Job drawing, mm, ordinate dimensions from the low corner. One solid piece. A direction names the side the tool comes from. Coordinates: 2 decimals unless noted, no trailing zeros. Write each loop counter-clockwise with the first axis right and the second up, starting at its lowest first coordinate (ties: lowest second). Pieces come first, ordered by that corner, then holes.
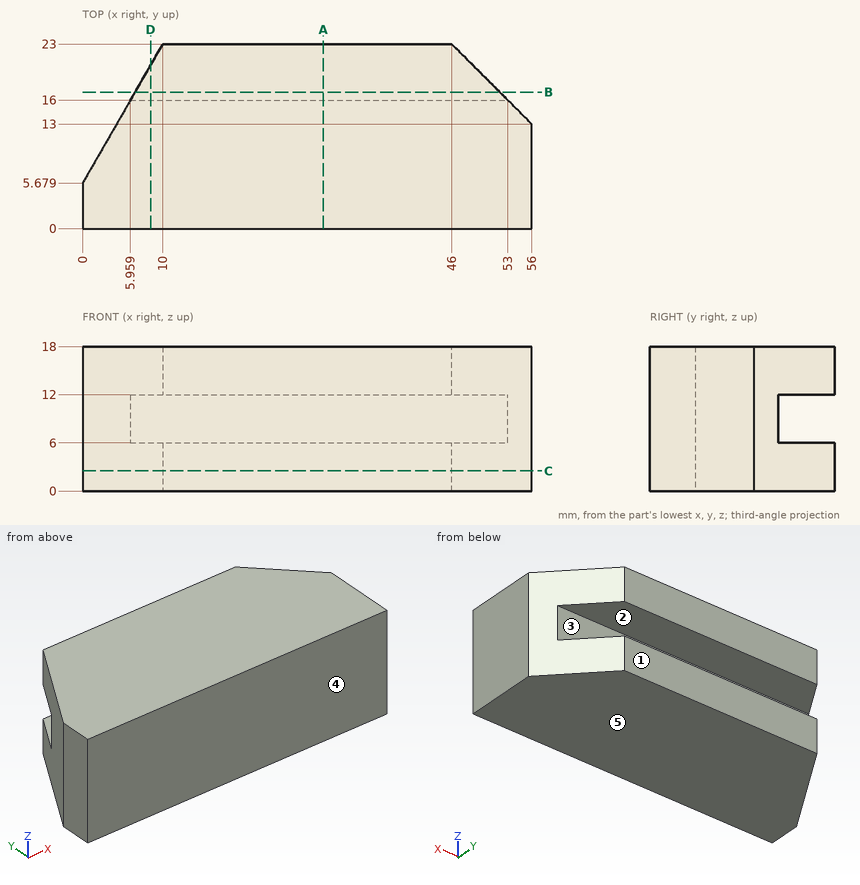
1. Saw through at D-D on x = 8.5. List the corners of the cut face in (y, z).
Computed values:
outline: (0, 0) - (20.4, 0) - (20.4, 6) - (16, 6) - (16, 12) - (20.4, 12) - (20.4, 18) - (0, 18) - close
2. 3-axis set-ups, long thin cutter, end or side, ignore diameter. For the marked faces 1 and 2: which of +Z, -Z, +X, -X, +Y, -Y reach the whole face in a straight line?
Computed values:
face 1: +Z, -Z, +X, -X, +Y
face 2: +X, -X, +Y
3. Saw through at A-A on x = 30. List the corners of the cut face in (y, z).
Computed values:
outline: (0, 0) - (23, 0) - (23, 6) - (16, 6) - (16, 12) - (23, 12) - (23, 18) - (0, 18) - close
4. Saw through at C-C on z = 2.5. List the corners of the cut face in (x, y).
Computed values:
outline: (0, 0) - (56, 0) - (56, 13) - (46, 23) - (10, 23) - (0, 5.68) - close
5. Flat gauge pins, fed straight in: pin 1 (6 mm diameter, centred on x = 10.5, z = 6.5, fed in from +Y); pin 2 (3 mm diameter, centred on x = 21.5, z = 10, fed in from +Y); pin 3 (3 mm diameter, centred on y = 16.5, z = 13, fed in from +X); pin 4 (5 mm diameter, centred on y = 20.5, z = 2, fed in from +X). Where does each tip first touch, or does it go through?
Computed values:
pin 1: stops at y = 23
pin 2: stops at y = 16
pin 3: stops at x = 54
pin 4: stops at x = 51
6. Probe line 1 along Z through (x, y) = (29.5, 19.25); line 2 along Y through (x, z) = (36, 6.75); line 3 along X through (y, z) = (20.5, 2) (1 decimal). List the from-to ranges inside material, lowest first.
Computed values:
line 1: z = 0 to 6, 12 to 18
line 2: y = 0 to 16
line 3: x = 8.6 to 48.5
7. Mould opens along Z. For the marked faces 3, 4 and 5 say: +Z half, -Z half, draft (parallel to the pull), parting line (faces both ways), or undercut.
Computed values:
face 3: undercut
face 4: draft
face 5: -Z half
8. Saw through at B-B on y = 17. List the corners of the cut face in (x, z) (1 decimal).
Computed values:
outline: (6.5, 0) - (52, 0) - (52, 6) - (6.5, 6) - close; (6.5, 12) - (52, 12) - (52, 18) - (6.5, 18) - close
